Read the model definition and answer for the solid it produces. Units are mm, in the model's axes. Give positions to 0.01 mm unless a question says otherwise; leave off trailing zeros. Order: outer loops, then holes, each group sorted by start corner. A loop starts at its lowest first (then second) coordinate and runs counter-clockwise, first axis right, second up. Notation, with made-up numbers: (89, 13.25) - (99, 13.25) arc R14 cw to (99, 36.25) - close; hole circle Ø9 at (55, 56). An arc over 180 degrees is marked (long way). Use a Markdown table: item, result. Add a question column.
1. Flat-ended cylindrical pins translate along their axes: P1, Ø1.5, axis at y = -23, z = 1.5, coming from the -X side; P2, Ø1.5, axis at x = -16.5, z = 1.5, coming from the +Y side; P3, Ø1.1, axis at y = 11.5, z = 2, coming from the +X side. Find the tip coordinate at first contact, or state that the pin passes through.
2. A cutting plane is placed at C-C on z = 1.8. State how many separate pieces and enclosed holes the cut face has, and give its area (3 significant figures).
3. A cutting plane is placed at A-A on y = -29. Determine the outline of the cut face in (x, z).
4. Consider L1, parallel to Y at x = 15, z = 2; L2, parallel to X at y = -4, z = 2.65; L3, parallel to Y at x = -12, z = 0.95. Determine where each line is inside the solid, lowest interval first.
5. A cutting plane is placed at B-B on y = -15.5. Determine the outline of the cut face in (x, z), and give its area (3 significant figures).
```python
from build123d import *

# Parameters (mm, degrees)
BOSS_EXTRUDE2_DEPTH = 4


with BuildPart() as part:
    # Sketch1 → Boss-Extrude2 (new body)
    # profile 1 of 2: a face of its own
    with BuildSketch(Plane.XY):
        with BuildLine():
            ThreePointArc((-18.10386699, -12.5), (-22, 0), (-18.10386699, 12.5))
            Line((-18.10386699, 12.5), (-80.44, 4.950136038))
            Line((-80.44, 4.950136038), (-92.44, 6))
            Line((-92.44, 6), (-92.44, -6))
            Line((-92.44, -6), (-80.44, -4.950136038))
            Line((-80.44, -4.950136038), (-18.10386699, -12.5))
        make_face()
    # profile 2 of 2: a face of its own
    with BuildSketch(Plane.XY):
        with BuildLine():
            ThreePointArc((0, 22), (4.39692325, 24.688021922), (7.624562296, 28.705576167))
            Line((7.624562296, 28.705576167), (28.576895981, 49.746134685))
            ThreePointArc((28.576895981, 49.746134685), (57.361992188, -0.958515634), (26.898895733, -50.673132016))
            Line((26.898895733, -50.673132016), (14.293358327, -23.788083824))
            ThreePointArc((14.293358327, -23.788083824), (7.375363605, -21.066013146), (0, -22))
            ThreePointArc((0, -22), (-22, 0), (0, 22))
        make_face()
        with BuildLine():
            ThreePointArc((-10.905276344, 1.44046793), (-10.461621679, -3.399186938), (-7.975868085, -7.575323642))
            Line((-7.975868085, -7.575323642), (-9.250831414, -9.330160117))
            ThreePointArc((-9.250831414, -9.330160117), (-8.816778784, -12.135254915), (-6.014845458, -11.681241534))
            Line((-6.014845458, -11.681241534), (-4.73988213, -9.926405059))
            ThreePointArc((-4.73988213, -9.926405059), (0, -11), (4.73988213, -9.926405059))
            Line((4.73988213, -9.926405059), (6.014845458, -11.681241534))
            ThreePointArc((6.014845458, -11.681241534), (8.816778784, -12.135254915), (9.250831414, -9.330160117))
            Line((9.250831414, -9.330160117), (7.975868085, -7.575323642))
            ThreePointArc((7.975868085, -7.575323642), (10.461621679, -3.399186938), (10.905276344, 1.44046793))
            Line((10.905276344, 1.44046793), (12.968210344, 2.110755818))
            ThreePointArc((12.968210344, 2.110755818), (14.265847744, 4.635254915), (11.732173696, 5.914885461))
            Line((11.732173696, 5.914885461), (9.669239696, 5.244597572))
            ThreePointArc((9.669239696, 5.244597572), (6.465637775, 8.899186938), (1.999949308, 10.816663199))
            Line((1.999949308, 10.816663199), (1.999949308, 12.985760372))
            ThreePointArc((1.999949308, 12.985760372), (0, 15), (-1.999949308, 12.985760372))
            Line((-1.999949308, 12.985760372), (-1.999949308, 10.816663199))
            ThreePointArc((-1.999949308, 10.816663199), (-6.465637775, 8.899186938), (-9.669239696, 5.244597572))
            Line((-9.669239696, 5.244597572), (-11.732173696, 5.914885461))
            ThreePointArc((-11.732173696, 5.914885461), (-14.265847744, 4.635254915), (-12.968210344, 2.110755818))
            Line((-12.968210344, 2.110755818), (-10.905276344, 1.44046793))
        make_face(mode=Mode.SUBTRACT)
        with BuildLine():
            ThreePointArc((20.173023673, -8.777762578), (21.622154849, 4.05985464), (15.61502008, 15.497456175))
            ThreePointArc((15.61502008, 15.497456175), (14.163890039, 19.023799586), (15.620934225, 22.547703457))
            Line((15.620934225, 22.547703457), (29.479774673, 36.464899881))
            ThreePointArc((29.479774673, 36.464899881), (32.923189008, 37.935810816), (36.42242793, 36.603141231))
            ThreePointArc((36.42242793, 36.603141231), (51.457765207, 2.212369547), (36.504075375, -32.213982342))
            ThreePointArc((36.504075375, -32.213982342), (32.145722027, -33.464647666), (28.568596515, -30.678327382))
            Line((28.568596515, -30.678327382), (20.230712329, -12.895315764))
            ThreePointArc((20.230712329, -12.895315764), (19.758292439, -10.842753852), (20.173023673, -8.777762578))
        make_face(mode=Mode.SUBTRACT)
    extrude(amount=BOSS_EXTRUDE2_DEPTH)


solid = part.part
```
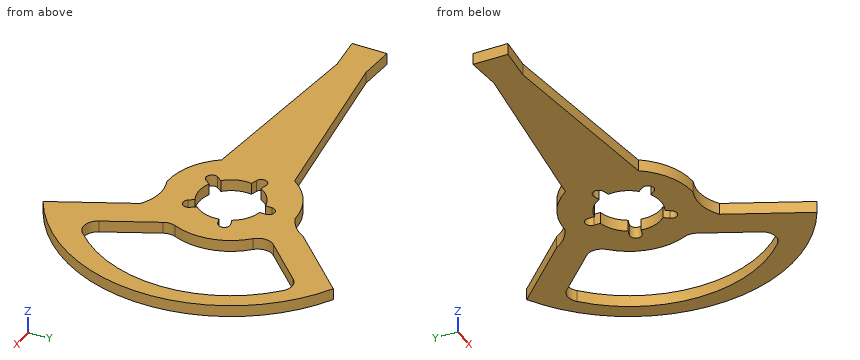
Output values:
| question | item | result |
|---|---|---|
| 1 | P1 | x = 11.62 |
| 1 | P2 | y = 15.36 |
| 1 | P3 | x = 56.32 |
| 2 | separate pieces | 1 |
| 2 | enclosed holes | 2 |
| 2 | area | 3,610 mm² |
| 3 | outline | (16.74, 0) - (27.78, 0) - (27.78, 4) - (16.74, 4) - close; (39.64, 0) - (49.5, 0) - (49.5, 4) - (39.64, 4) - close |
| 4 | L1 | -25.3 to 16.25, 21.79 to 36.11 |
| 4 | L2 | -92.44 to -10.25, 10.25 to 21.63, 51.05 to 57.23 |
| 4 | L3 | -18.44 to 1.8, 5.98 to 18.44 |
| 5 | outline | (-15.61, 0) - (21.45, 0) - (21.45, 4) - (-15.61, 4) - close; (48.01, 0) - (55.24, 0) - (55.24, 4) - (48.01, 4) - close |
| 5 | area | 177 mm² |
